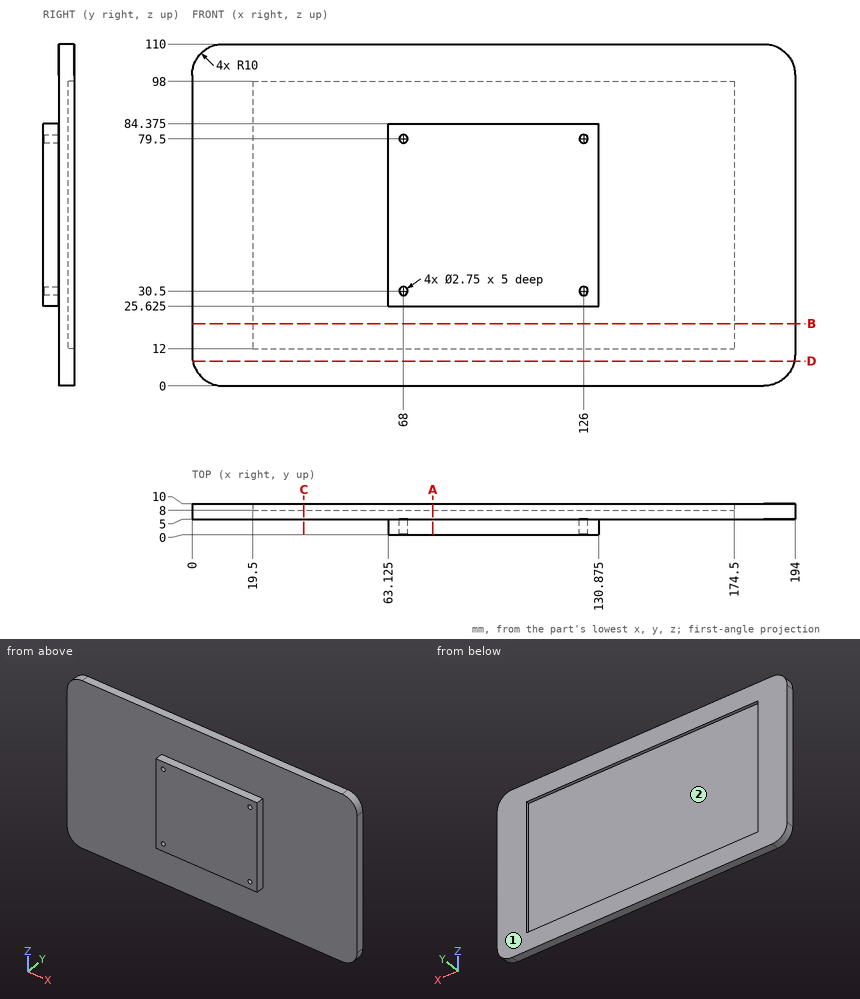
Can you work these out from the drawing? Everything is in mm from the part's minimum corner. Round coordinates to 2 decimals unless told otherwise and drop trailing zeros. Loops run counter-clockwise (first coordinate to the right, second up) from the corner with the lowest first, then second, coordinate; pieces in that order, holes last. Notation, with made-up numbers: M 55,86 L 89,86 A15 cw 89,112 Z; hole C -18,31 d6. An arc over 180 degrees is marked long. Answer in a Markdown table with one row per item.
1. If we section it at D-D, the plane z = 8: Please give me the cut outline in (x, y), plus the area to 3 significant figures.
Established:
| item | result |
|---|---|
| outline | M 0.2,5 L 193.8,5 L 193.8,10 L 0.2,10 Z |
| area | 968 mm² |
2. If we section it at C-C, the plane x = 36: Please give me the cut outline in (y, z), plus the area to 3 significant figures.
Established:
| item | result |
|---|---|
| outline | M 5,0 L 10,0 L 10,12 L 8,12 L 8,98 L 10,98 L 10,110 L 5,110 Z |
| area | 378 mm² |
3. If we section it at B-B, the plane z = 20: Please give me the cut outline in (x, y).
Established:
| item | result |
|---|---|
| outline | M 0,5 L 194,5 L 194,10 L 174.5,10 L 174.5,8 L 19.5,8 L 19.5,10 L 0,10 Z |
4. Thinking about a two-plate mould opening in Z: for the marked faces 1 and 2, which applies, pulls with the +Z half, pulls with the -Z half, needs draft (parallel to the pull), parting line crosses it, or undercut?
Established:
| item | result |
|---|---|
| face 1 | needs draft |
| face 2 | undercut |
5. If we section it at A-A, the plane x = 77.5: Please give me the cut outline in (y, z) (3 decimals).
Established:
| item | result |
|---|---|
| outline | M 0,25.625 L 5,25.625 L 5,0 L 10,0 L 10,12 L 8,12 L 8,98 L 10,98 L 10,110 L 5,110 L 5,84.375 L 0,84.375 Z |
6. Please list where these lines run through material, in increasing order: line 1 (X direction, y = 2.85, z = 30.5) (3 decimals); line 2 (X direction, y = 8.5, z = 16); line 3 (Z direction, x = 163, y = 9.75). Write a range as from..to.
Established:
| item | result |
|---|---|
| line 1 | 63.125..66.625, 69.375..124.625, 127.375..130.875 |
| line 2 | 0..19.5, 174.5..194 |
| line 3 | 0..12, 98..110 |
7. I'm going to push flat-ended pins straight in: pin 1 Ø12 at (x, z) = (165.5, 61) entering from -Y; pin 2 Ø4 at (x, y) = (81, 3.5) entering from -Z; pin 3 Ø3 at (x, z) = (126, 30.5) entering from +Y; pin 4 Ø2 at (y, z) = (2.5, 48) entering from +X (3 decimals). Where does each tip first touch, or does it pass through?
Established:
| item | result |
|---|---|
| pin 1 | y = 5 |
| pin 2 | z = 0 |
| pin 3 | y = 8 |
| pin 4 | x = 130.875 |
